The model under review builds one solid part; all positions refer to its coordinate system, in mm. Face numbers are marked on the shaded views. Coordinates: 2 decimals unless noted, no trailing zeros. Loops run counter-clockwise (first coordinate to the right, second up) from the corner with the lowest first, then second, coordinate; pieces in that order, holes last. Notation, with made-up numbers: (17, 73) - (54, 73) arc R24 ccw to (54, 84) - close; hole circle Ø10 at (55, 57). An arc over 180 degrees is marked (long way). Use a Markdown table: item, result. Add a question column.
1) Add section A-A, the plane z = 3.05. Give the number of separate pieces and of enclosed holes in the cut face, and give its area (3 significant figures).
2) Add section C-C, the plane y = 3. Give the boundary of the cut face in (x, z), and give its area (3 significant figures).
3) The part is to be moulded in two halves that separate along X. For the marked faces 1, 2, 3 and 4, say which applies: pulls with the +X half, pulls with the -X half, needs draft (parallel to the pull), parting line crosses it, or undercut.
4) Clearance check with flat-ended pins moving along their axes: pin 1 (1.8 mm diameter, centred on x = -23.12, y = -19.37, fed in from +Z); pin 2 (1.5 mm diameter, centred on y = -8, z = 1, fed in from -X); pin 3 (1.7 mm diameter, centred on x = -15.5, y = -27, fed in from -Z). State where each tip first meets the part, or that it passes through.
5) To check wall thickness, follow L1, parallel to Y at x = -15.25, z = 1.55; L2, parallel to Y at x = -21.25, z = 3.85; L3, parallel to Y at x = -8.25, z = 0.5. State the ranges of each line that lie inside material, in increasing order. Write a range as [from, to].
```python
from build123d import *

# Parameters (mm, degrees)
SKETCH1_R           = 1.55
SKETCH1_R_2         = 4.25
SKETCH1_R_3         = 1.1
BOSS_EXTRUDE1_DEPTH = 5
CUT_EXTRUDE2_DEPTH  = 2
SKETCH4_R           = 1.75
CUT_EXTRUDE3_DEPTH  = 2.25
CHAFL_N1_SIZE       = 0.75


with BuildPart() as part:
    # Sketch1 → Boss-Extrude1 (new body)
    with BuildSketch(Plane.XY):
        with BuildLine():
            Line((-23.088186689, 16.318953541), (-26.077145964, -18.423903602))
            ThreePointArc((-26.077145964, -18.423903602), (-15.11762862, -30.366760745), (-4.158111277, -18.423903602))
            Line((-4.158111277, -18.423903602), (-7.147070552, 16.318953541))
            ThreePointArc((-7.147070552, 16.318953541), (-15.11762862, 23.633239255), (-23.088186689, 16.318953541))
        make_face()
        with Locations((-15.11762862, 15.633239255)):
            Circle(SKETCH1_R, mode=Mode.SUBTRACT)
        with Locations((-15.11762862, -19.366760745)):
            Circle(SKETCH1_R_2, mode=Mode.SUBTRACT)
        with Locations((-7.11762862, -19.366760745)):
            Circle(SKETCH1_R_3, mode=Mode.SUBTRACT)
        with Locations((-9.460774371, -25.023614994)):
            Circle(SKETCH1_R_3, mode=Mode.SUBTRACT)
        with Locations((-15.11762862, -27.366760745)):
            Circle(SKETCH1_R_3, mode=Mode.SUBTRACT)
        with Locations((-20.77448287, -25.023614994)):
            Circle(SKETCH1_R_3, mode=Mode.SUBTRACT)
        with Locations((-23.11762862, -19.366760745)):
            Circle(SKETCH1_R_3, mode=Mode.SUBTRACT)
        with Locations((-20.77448287, -13.709906495)):
            Circle(SKETCH1_R_3, mode=Mode.SUBTRACT)
        with Locations((-15.11762862, -11.366760745)):
            Circle(SKETCH1_R_3, mode=Mode.SUBTRACT)
        with Locations((-9.460774371, -13.709906495)):
            Circle(SKETCH1_R_3, mode=Mode.SUBTRACT)
    extrude(amount=BOSS_EXTRUDE1_DEPTH)

    # Sketch3 → Cut-Extrude2 (cut)
    with BuildSketch(Plane.XY):
        Polygon((-13.52991538, 12.883239255), (-11.94220214, 15.633239255), (-13.52991538, 18.383239255), (-16.705341861, 18.383239255), (-18.293055101, 15.633239255), (-16.705341861, 12.883239255), align=None)
    extrude(amount=CUT_EXTRUDE2_DEPTH, mode=Mode.SUBTRACT)

    # Sketch4 → Cut-Extrude3 (cut)
    with BuildSketch(Plane(origin=(0, 0, 0), x_dir=(-1, 0, 0), z_dir=(0, 0, -1))):
        with Locations((23.11762862, -19.366760745)):
            Circle(SKETCH4_R)
        with Locations((20.77448287, -25.023614994)):
            Circle(SKETCH4_R)
        with Locations((15.11762862, -27.366760745)):
            Circle(SKETCH4_R)
        with Locations((9.460774371, -25.023614994)):
            Circle(SKETCH4_R)
        with Locations((7.11762862, -19.366760745)):
            Circle(SKETCH4_R)
        with Locations((9.460774371, -13.709906495)):
            Circle(SKETCH4_R)
        with Locations((15.11762862, -11.366760745)):
            Circle(SKETCH4_R)
        with Locations((20.77448287, -13.709906495)):
            Circle(SKETCH4_R)
    extrude(amount=-CUT_EXTRUDE3_DEPTH, mode=Mode.SUBTRACT)

    # Chaflán1
    chafl_n1_edges = [part.edges().sort_by_distance(p)[0] for p in [
        (-5.652590914, -1.05247503, 0),
        (-15.11762862, -30.366760745, 0),
        (-24.582666326, -1.05247503, 0),
        (-15.11762862, 23.633239255, 0),
    ]]
    chamfer(chafl_n1_edges, length=CHAFL_N1_SIZE)


solid = part.part
```
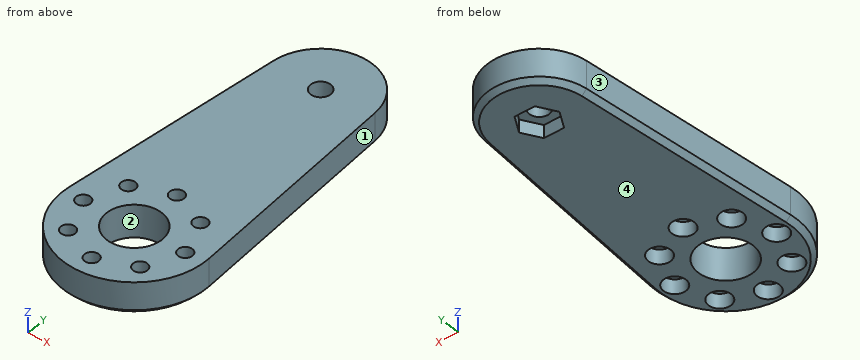
From the geometry:
| question | item | result |
|---|---|---|
| 1 | separate pieces | 1 |
| 1 | enclosed holes | 10 |
| 1 | area | 863 mm^2 |
| 2 | outline | (-24.23, 0.75) - (-23.48, 0) - (-6.75, 0) - (-6, 0.75) - (-6, 5) - (-24.23, 5) - close |
| 2 | area | 90.6 mm^2 |
| 3 | face 1 | pulls with the +X half |
| 3 | face 2 | undercut |
| 3 | face 3 | pulls with the -X half |
| 3 | face 4 | needs draft |
| 4 | pin 1 | passes through |
| 4 | pin 2 | stops at x = -25.24 |
| 4 | pin 3 | stops at z = 2.25 |
| 5 | L1 | y = [-30.37, -29.11], [-25.62, -23.61], [-15.12, -13.11], [-9.62, 12.88], [18.38, 23.63] |
| 5 | L2 | y = [-28.5, -26.02], [-24.03, -14.7], [-12.72, 20.77] |
| 5 | L3 | y = [-27.64, -26.29], [-23.76, -20.7], [-18.03, -14.97], [-12.45, 19.22] |
